Build history of the part. All positions in model axes, mm. A direction names the side the tool comes from. Give positions to 0.01 mm unless a question says otherwise; leave off trailing zeros. Order: outer loops, then holes, each group sorted by start corner. A loop starts at its lowest first (then second) coordinate and runs counter-clockwise, first axis right, second up. Notation, with made-up numbers: (38, 5.5) - (43, 5.5) arc R28 cw to (43, 24.5) - close; hole circle Ø6 at (-21, 17). An arc over 180 degrees is marked (long way). Use a Markdown table: item, result.
from build123d import *

# Parameters (mm, degrees)
F1_DEPTH = 0.508
F2_W     = 65.868683
F2_H     = 1.016
F3_DEPTH = 0.509


with BuildPart() as f1:
    # F0 (on Front) → F1 (new body)
    with BuildSketch(Plane.XZ):
        with BuildLine():
            Line((39.37, 25.4), (-39.37, 25.4))
            ThreePointArc((-39.37, 25.4), (-42.962102, 23.912102), (-44.45, 20.32))
            Line((-44.45, 20.32), (-44.45, -20.32))
            ThreePointArc((-44.45, -20.32), (-42.962102, -23.912102), (-39.37, -25.4))
            Line((-39.37, -25.4), (39.37, -25.4))
            ThreePointArc((39.37, -25.4), (42.962102, -23.912102), (44.45, -20.32))
            Line((44.45, -20.32), (44.45, 20.32))
            ThreePointArc((44.45, 20.32), (42.962102, 23.912102), (39.37, 25.4))
        make_face()
    extrude(amount=F1_DEPTH)

    # F2 (on face) → F3 (cut, through all)
    with BuildSketch(Plane.XZ.offset(0.508)):
        Polygon((-24.913168, 10.547717), (-10.842625, -1.23167), (-19.243895, -11.267034), (35.490545, -11.267034), (35.490545, -20.32), (36.506545, -20.32), (36.506545, -10.251034), (-17.068302, -10.251034), (-9.411394, -1.104816), (-25.040023, 11.978947), (-38.123786, -3.649681), (-35.458138, -5.881272), (-35.458138, -20.32), (-34.442138, -20.32), (-34.442138, -5.406801), (-36.692555, -3.522827), align=None)
        with Locations((0.524204, -19.812)):
            Rectangle(F2_W, F2_H)
    extrude(amount=-F3_DEPTH, mode=Mode.SUBTRACT)


solid = f1.part
1) Slice it at A-A (y = -0.15). Write the cut outline in (x, z).
Computed:
| item | result |
|---|---|
| outline | (-44.45, -20.32) arc R5.08 ccw to (-39.37, -25.4) - (39.37, -25.4) arc R5.08 ccw to (44.45, -20.32) - (44.45, 20.32) arc R5.08 ccw to (39.37, 25.4) - (-39.37, 25.4) arc R5.08 ccw to (-44.45, 20.32) - close; hole (-38.12, -3.65) - (-35.46, -5.88) - (-35.46, -20.32) - (-34.44, -20.32) - (-34.44, -5.41) - (-36.69, -3.52) - (-24.91, 10.55) - (-10.84, -1.23) - (-19.24, -11.27) - (35.49, -11.27) - (35.49, -20.32) - (36.51, -20.32) - (36.51, -10.25) - (-17.07, -10.25) - (-9.41, -1.1) - (-25.04, 11.98) - close; hole (-32.41, -20.32) - (33.46, -20.32) - (33.46, -19.3) - (-32.41, -19.3) - close |
2) Wall check: line 1 (X direction, y = -0.4, z = -12); line 2 (Z direction, x = 33, y = -0.4); line 3 (X direction, y = -0.1, z = -19.5). Give the ranges that are in metal, low to high. Write a range as from..to.
Computed:
| item | result |
|---|---|
| line 1 | x = -44.45..-35.46, -34.44..35.49, 36.51..44.45 |
| line 2 | z = -25.4..-20.32, -19.3..-11.27, -10.25..25.4 |
| line 3 | x = -44.45..-35.46, -34.44..-32.41, 33.46..35.49, 36.51..44.45 |
3) Tool access for faces 1 (the flat face through (-13.29, -0.26, -5.74)), 2 (the flat face through (-1, -0.508, 0)): list every direction of +Z, -Z, +X, -X, +Y, -Y with a clear straight run to the whole face (end or side of a thin tool).
Computed:
| item | result |
|---|---|
| face 1 | +Y, -Y |
| face 2 | +Z, -Z, +X, -X, -Y |
4) Pin check, flat tip, straight feed: P1, Ø3, axis at x = 25.5, z = 19.5, coming from the +Y side. Stop position of the tip, or through.
Computed:
| item | result |
|---|---|
| P1 | stops at y = 0 |
5) Slice it at D-D (x = -15.5). Write the cut outline in (y, z), and give its area (3 significant figures).
Computed:
| item | result |
|---|---|
| outline | (-0.51, -25.4) - (0, -25.4) - (0, -20.32) - (-0.51, -20.32) - close; (-0.51, -19.3) - (0, -19.3) - (0, -11.27) - (-0.51, -11.27) - close; (-0.51, -10.25) - (0, -10.25) - (0, -8.38) - (-0.51, -8.38) - close; (-0.51, -6.79) - (0, -6.79) - (0, 2.67) - (-0.51, 2.67) - close; (-0.51, 3.99) - (0, 3.99) - (0, 25.4) - (-0.51, 25.4) - close |
| area | 23.3 mm² |
6) Slice it at C-C (x = 3). Write the cut outline in (y, z), and give its area (3 significant figures).
Computed:
| item | result |
|---|---|
| outline | (-0.51, -25.4) - (0, -25.4) - (0, -20.32) - (-0.51, -20.32) - close; (-0.51, -19.3) - (0, -19.3) - (0, -11.27) - (-0.51, -11.27) - close; (-0.51, -10.25) - (0, -10.25) - (0, 25.4) - (-0.51, 25.4) - close |
| area | 24.8 mm² |
7) Two-plate mould, pull along X, no slides. Class faces 3 (the flat face through (-1, 0, 0)), 4 (the flat face through (-15, -0.3, -6.2)), 5 (the cylindrical face through (42.922, -0.25, -23.951)): +X half, -X half, draft (parallel to the pull), parting line (faces both ways), or undercut.
Computed:
| item | result |
|---|---|
| face 3 | draft |
| face 4 | undercut |
| face 5 | +X half |
8) Slice it at B-B (z = -18). Write the cut outline in (x, y), and give its area (3 significant figures).
Computed:
| item | result |
|---|---|
| outline | (-44.45, -0.51) - (-35.46, -0.51) - (-35.46, 0) - (-44.45, 0) - close; (-34.44, -0.51) - (35.49, -0.51) - (35.49, 0) - (-34.44, 0) - close; (36.51, -0.51) - (44.45, -0.51) - (44.45, 0) - (36.51, 0) - close |
| area | 44.1 mm² |
